The model under review builds one solid part; all positions refer to its coordinate system, in mm. Round coordinates to 2 decimals unless told otherwise and drop trailing zeros. Write each loop counter-clockwise with the first axis right and the second up, starting at its lowest first coordinate (ties: lowest second). Pieces come first, ordered by that corner, then holes. Notation, with made-up numbers: (-33, -15.5) -> (-26, -15.5) arc R30 cw to (-26, 20.5) -> close; hole circle Ø8 at (55, -19.75). An arc over 180 degrees is marked (long way). Answer in a Markdown table with one row per item. Add a question column.
Autodesk Inventor part; units mm, degrees
ref_plane "YZ Plane" through (0, 0, 0) normal (1, 0, 0) x (0, 1, 0)
ref_plane "XZ Plane" through (0, 0, 0) normal (0, 1, 0) x (-1, 0, 0)
ref_plane "XY Plane" through (0, 0, 0) normal (0, 0, 1) x (1, 0, 0)
sketch "Sketch1" plane through (0, 0, 0) normal (0, 0, 1) x (1, 0, 0)
  circle A0 centre (24.0765, 0.0001) radius 15
  point P0 (0, 0)
  dimension "d0" = 30
extrude "Extrusion1" add sketch "Sketch1" along normal blind 3.5
chamfer "Chamfer1" distance 3 distance2 5 1 edges at (9.0765, 0.0001, 3.5) measured on face at (38.8822, -2.4061, 2.3333)
chamfer "Chamfer2" distance 0.25 angle 45 1 edges at (9.0765, 0.0001, 0)
sketch "Sketch2" plane through (24.0765, 0.0001, 3.5) normal (0, 0, 1) x (1, 0, 0)
  circle A0 centre (0, 0) radius 10
  circle A1 centre (0, 0) radius 9.25
  point P0 (-24.0765, -0.0001)
  dimension "d9" = 18.5
extrude "Extrusion2" cut sketch "Sketch2" against normal blind 0.65 contours A1
fillet "Fillet2" radius 2 2 edges at (14.8265, 0.0001, 3.5) (14.0765, 0.0001, 3.5)
sketch "Sketch3" plane through (24.0765, 0.0001, 2.85) normal (0, 0, 1) x (1, 0, 0)
  circle A0 centre (0, 0) radius 9.25
  point P0 (-24.0765, -0.0001)
extrude "Extrusion3" cut sketch "Sketch3" against normal through all
properties part number "objektiv"
1. Add section A-A on z = 2.3. Write out the cut boundary in (x, y).
2. For L1, parallel to Y at x = 21, z = 2.6; L2, parallel to Y at x = 23, z = 2.65; L3, parallel to X at y = -1.5, z = 1.4, list the stretches that pass through material, from the lowest coordinate up.
3. Mouldability with a two-part tool opening along X and no side actions: class faces 1 (the conical face through (34.635, 4.378, 2.642)), 2 (the cylindrical face through (14.835, 0.407, 1.445)), 3 (the flat face through (34, 0, 0)) as pulls with the +X half, pulls with the -X half, needs draft (parallel to the pull), parting line crosses it, or undercut.
Filled in:
| question | item | result |
|---|---|---|
| 1 | outline | circle Ø24 at (24.08, 0); hole circle Ø18.5 at (24.08, 0) |
| 2 | L1 | -11.08 to -8.72, 8.72 to 11.08 |
| 2 | L2 | -11.37 to -9.19, 9.19 to 11.37 |
| 2 | L3 | 10.66 to 14.95, 33.2 to 37.49 |
| 3 | face 1 | parting line crosses it |
| 3 | face 2 | undercut |
| 3 | face 3 | needs draft |
